Study the drawing (mm; zero at the part's minimum x, y, z) and answer. A direction names the side the tool comes from. Coordinates: 2 decimals unless noted, no trailing zeros. Order: outer loops, then holes, each group sorted by start corner. A loop starts at its lowest first (then second) coordinate and runs counter-clockwise, first axis right, second up. Notation, with made-up numbers: (84.25, 19) - (118.25, 19) arc R30 cw to (118.25, 51) - close; hole circle Ø9 at (10, 56.5). An arc over 180 degrees is marked (long way). Write item = value, one per line.
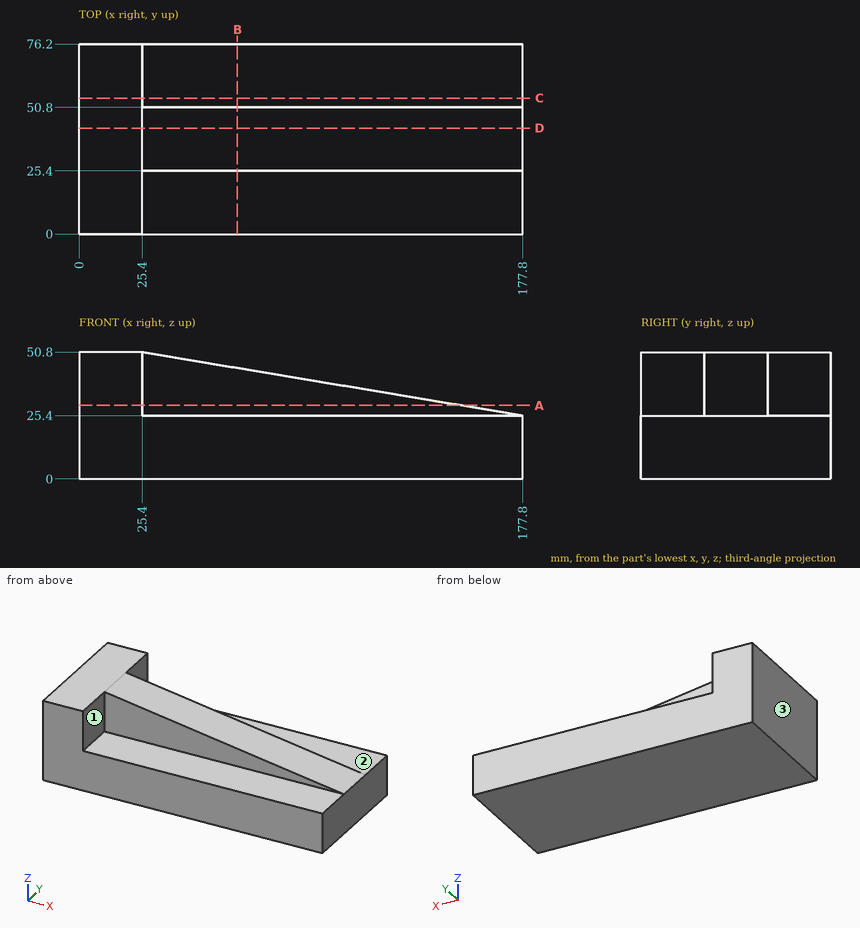
1) The part is cut by section D-D (y = 42.5). Determine the outline of the cut face in (x, z), and give its area (3 significant figures).
Returned:
outline = (0, 0) - (177.8, 0) - (177.8, 25.4) - (25.4, 50.8) - (0, 50.8) - close
area = 7,100 mm^2
2) The part is cut by section C-C (y = 54.5). Determine the outline of the cut face in (x, z).
Returned:
outline = (0, 0) - (177.8, 0) - (177.8, 25.4) - (25.4, 25.4) - (25.4, 50.8) - (0, 50.8) - close
3) The part is cut by section A-A (z = 29.5). Determine the outline of the cut face in (x, y).
Returned:
outline = (0, 0) - (25.4, 0) - (25.4, 25.4) - (153.2, 25.4) - (153.2, 50.8) - (25.4, 50.8) - (25.4, 76.2) - (0, 76.2) - close
4) Flat-ended cylindrical pins translate along their axes: pin 1 Ø1.5 at (y, z) = (59, 42.5) entering from +X; pin 2 Ø7.5 at (x, z) = (120.5, 33) entering from +Y; pin 3 Ø1.5 at (x, z) = (87, 37) entering from -Y. Find the tip coordinate at first contact, or state that the pin passes through.
Returned:
pin_1 = 25.4
pin_2 = 50.8
pin_3 = 25.4
5) For the marked faces 1, 2 and 3, determine the directions among +Z, -Z, +X, -X, +Y, -Y from which every point of the face is accessible in a straight line to the end or side of a thin tool.
Returned:
face_1 = +Z, +X, -Y
face_2 = +Z, +X, +Y
face_3 = +Z, -Z, -X, +Y, -Y
6) Straight lines are drawn through the part: line 1 along Z through (x, y) = (153, 65.5); line 2 along Y through (x, z) = (31.5, 38.5). For each, find the intervals that lie inside material, in ascending order. Write a range as from..to.
Returned:
line_1 = 0..25.4
line_2 = 25.4..50.8
7) The part is cut by section B-B (x = 63.5). Determine the outline of the cut face in (y, z), and give its area (3 significant figures).
Returned:
outline = (0, 0) - (76.2, 0) - (76.2, 25.4) - (50.8, 25.4) - (50.8, 44.45) - (25.4, 44.45) - (25.4, 25.4) - (0, 25.4) - close
area = 2,420 mm^2
